from build123d import *

# Parameters (mm, degrees)
F0_W     = 175
F0_H     = 100
F1_DEPTH = 85
F2_R     = 49.99999
F3_R     = 49.99999
F6_R     = 2.4206343252
F7_DEPTH = 15.2
F8_R     = 2.136311852
F9_DEPTH = 121.8


# Not quite as in the source:
# - a fillet or chamfer is up to 0.001 mm smaller than in the source, because OpenCascade refuses the exact size
# - the program builds the solid bodies; features that only make, move or delete a surface that nothing else refers to are left out


with BuildPart() as f1:
    # F0 (on Top) → F1 (new body)
    with BuildSketch(Plane.XY):
        with Locations((87.5, 50)):
            Rectangle(F0_W, F0_H)
    extrude(amount=F1_DEPTH)

    # F2 (radius 50 in the source; OpenCascade refuses exactly that, so slightly less here)
    f2_edges = [f1.edges().sort_by_distance(p)[0] for p in [
        (0, 0, 42.5),
        (0, 100, 42.5),
    ]]
    fillet(f2_edges, radius=F2_R)

    # F3 (radius 50 in the source; OpenCascade refuses exactly that, so slightly less here)
    f3_edges = [f1.edges().sort_by_distance(p)[0] for p in [
        (175, 100, 42.5),
        (175, 0, 42.5),
    ]]
    fillet(f3_edges, radius=F3_R)

    # F6 (on face) → F7 (join)
    with BuildSketch(Plane(origin=(0, 0, 0), x_dir=(1, 0, 0), z_dir=(0, 0, -1))):
        with Locations((111.062400043, -6.450037472)):
            Circle(F6_R)
    extrude(amount=F7_DEPTH)

    # F8 (on face) → F9 (join)
    with BuildSketch(Plane(origin=(0, 0, 0), x_dir=(1, 0, 0), z_dir=(0, 0, -1))):
        with Locations((104.4254601002, -6.2192697078)):
            Circle(F8_R)
    extrude(amount=F9_DEPTH)


solid = f1.part
Source: CAD feature listing. Evaluate the final solid. Frame: model axes, mm. A direction names the side the tool comes from. Round coordinates to 2 decimals unless told otherwise and drop trailing zeros. Loops run counter-clockwise (first coordinate to the right, second up) from the corner with the lowest first, then second, coordinate; pieces in that order, holes last. Notation, with made-up numbers: (51, 15) - (96, 15) arc R21 ccw to (96, 25) - close; hole circle Ø6 at (37.25, 43.25). An arc over 180 degrees is marked (long way). Write item = value, one per line. Start each with the question number.
Item 1: Section query D-D on z = -49. Output: boundary loops of the cut face in (x, y), plus the area to 3 significant figures.
Item 2: Reachability of faces 1 (the face through (87, 0, 42)), 2 (the face through (111, 6, -15.2)) from +Z, -Z, +X, -X, +Y, -Y: full face, straight path, thin tool, end or side. Return the list, or none.
Item 3: First-contact query: pin 1 Ø5 at (x, y) = (42, 43) entering from -Z; pin 2 Ø5 at (y, z) = (73, 33.5) entering from +X; pin 3 Ø1.5 at (x, y) = (111, 6) entering from -Z. Flat tips, straight axial feed; report the tip coordinate or a pass-through.
Item 4: Mould query, pull axis X, two halves, no side actions, for faces 3 (the face through (86, 51, 85)), 4 (the face through (14.258, 15.036, 43.095)), 5 (the face through (113.37, 5.72, -7.49)). Classes: released by +X, released by -X, zero draft, split by the parting line, or undercut.
Item 5: Section query B-B on x = 68. Output: boundary loops of the cut face in (y, z), plus the area to 3 significant figures.
Item 6: Section query C-C on y = 64. Output: boundary loops of the cut face in (x, z), plus the area to 3 significant figures.
Item 7: Material intervals for line 1 (Z direction, x = 123, y = 15); line 2 (X direction, y = 48.5, z = 58); line 3 (X direction, y = 5, z = -3), sorted ascending.
Results list:
q1.outline = circle Ø4.27 at (104.43, 6.22)
q1.area = 14.3 mm²
q2.face_1 = +Z, -Z, +X, -X, -Y
q2.face_2 = -Z, +X, +Y, -Y
q3.pin_1 = 0
q3.pin_2 = 170.6
q3.pin_3 = -15.2
q4.face_3 = zero draft
q4.face_4 = released by -X
q4.face_5 = undercut
q5.outline = (0, 0) - (100, 0) - (100, 85) - (0, 85) - close
q5.area = 8,500 mm²
q6.outline = (2, 0) - (173, 0) - (173, 85) - (2, 85) - close
q6.area = 14,500 mm²
q7.line_1 = 0 to 85
q7.line_2 = 0.02 to 174.98
q7.line_3 = 102.67 to 106.18, 109.12 to 113
